Read the model definition and answer for the solid it produces. Units are mm, in the model's axes. A direction names the side the tool comes from. Round coordinates to 2 decimals unless told otherwise and drop trailing zeros. Write each loop counter-clockwise with the first axis right and the second up, starting at its lowest first coordinate (ties: lowest second). Pieces come first, ordered by that corner, then holes. Notation, with made-up numbers: (-30.5, 55) - (-8.5, 55) arc R26 cw to (-8.5, 94) - close; hole circle Ø3 at (55.5, 60.25). An arc over 180 degrees is marked (long way). One line per item, written item: value. Start each with the question number.
(1) A cutting plane is placed at A-A, the plane x = -27.8. Determine the outline of the cut face in (y, z).
(2) Find the intervals of material crossed by L1, parallel to X at y = 33, z = 96.5, in increasing order.
(3) For faces 1 (the face through (-27.76, 72.75, 2.54)), 2 (the face through (-18, 67, 5)), 3 (the face through (-18, 91, 5)), 4 (the face through (-5, 3, 179)), 5 (the face through (-5, 5, 91)), determine the directions among +Z, -Z, +X, -X, +Y, -Y from which every point of the face is accessible in a straight line to the end or side of a thin tool.
(4) A cutting plane is placed at C-C, the plane z = 120.5. Determine the outline of the cut face in (x, y).
(5) A cutting plane is placed at B-B, the plane x = -5. Determine the outline of the cut face in (y, z), plus the area to 3 significant figures.
(6) The mould has two halves that part along Y. Classify faces 6 (the face through (-10, 99, 3)), 7 (the face through (-3, 3, 175)), 8 (the face through (-29.55, 69, 3)): +Y half, -Y half, draft (parallel to the pull), parting line (faces both ways), or undercut.
(7) Flat-ended cylindrical pins translate along their axes: pin 1 Ø1.2 at (y, z) = (1.5, 58) entering from -X; pin 2 Ø8 at (x, z) = (-9, 80.5) entering from +Y; pin 3 Ø5 at (x, y) = (-19, 94.5) entering from +Z; pin 4 Ø12 at (x, z) = (-21.5, 145.5) entering from +Y. Find the tip coordinate at first contact, or state that the pin passes through.
(8) A cutting plane is placed at D-D, the plane x = -17. Determine the outline of the cut face in (y, z), plus the area to 3 significant figures.
from build123d import *

# Parameters (mm, degrees)
F0_W        = 54
F0_H        = 5
F0_W_2      = 40
F1_DEPTH    = 5
F2_DEPTH    = 10
F3_DEPTH    = 35
F5_DEPTH    = 5.001
F7_DEPTH    = 5.001
F4_W        = 35
F4_H        = 4
F8_DEPTH    = 40
F9_T4_DEPTH = 106.8673195186
F10_R       = 2
F11_R       = 10
F12_SIZE    = 0.6


# Not quite as in the source:
# - a fillet or chamfer that OpenCascade refuses, or shapes differently, is made with other operations: its cross-section is extruded or revolved along the edge and cut away or added


with BuildPart() as f1:
    # F0 (on Right) → F1 (new body)
    with BuildSketch(Plane.YZ):
        Polygon((0, 185), (0, 0), (5, 0), (5, 5), (5, 185), align=None)
        with Locations((32, 2.5)):
            Rectangle(F0_W, F0_H)
        Polygon((10, 185), (5, 185), (5, 5), (59, 5), (99, 5), (99, 10), align=None)
        with Locations((79, 2.5)):
            Rectangle(F0_W_2, F0_H)
    extrude(amount=F1_DEPTH)

    # F0 (on Right) → F2 (join)
    with BuildSketch(Plane.YZ):
        Polygon((0, 185), (0, 0), (5, 0), (5, 5), (5, 185), align=None)
    extrude(amount=-F2_DEPTH)

    # F0 (on Right) → F3 (join)
    with BuildSketch(Plane.YZ):
        with Locations((79, 2.5)):
            Rectangle(F0_W_2, F0_H)
    extrude(amount=-F3_DEPTH)

    # F4 (on face) → F5 (cut, through all)
    with BuildSketch(Plane.XY.offset(5)):
        with BuildLine():
            Line((-26.05, 69), (-26.05, 71))
            ThreePointArc((-26.05, 71), (-27.8, 72.75), (-29.55, 71))
            Line((-29.55, 71), (-29.55, 69))
            Line((-29.55, 69), (-29.55, 67))
            ThreePointArc((-29.55, 67), (-27.8, 65.25), (-26.05, 67))
            Line((-26.05, 67), (-26.05, 69))
        make_face()
        with BuildLine():
            Line((-26.05, 89), (-26.05, 91))
            ThreePointArc((-26.05, 91), (-27.8, 92.75), (-29.55, 91))
            Line((-29.55, 91), (-29.55, 89))
            Line((-29.55, 89), (-29.55, 87))
            ThreePointArc((-29.55, 87), (-27.8, 85.25), (-26.05, 87))
            Line((-26.05, 87), (-26.05, 89))
        make_face()
    extrude(amount=-F5_DEPTH, mode=Mode.SUBTRACT)

    # F6 (on face) → F7 (cut, through all)
    with BuildSketch(Plane(origin=(0, 5, 0), x_dir=(-1, 0, 0), z_dir=(0, 1, 0))):
        with BuildLine():
            Line((7, 58), (7, 60))
            ThreePointArc((7, 60), (5, 62), (3, 60))
            Line((3, 60), (3, 58))
            Line((3, 58), (3, 56))
            ThreePointArc((3, 56), (5, 54), (7, 56))
            Line((7, 56), (7, 58))
        make_face()
        with BuildLine():
            Line((7, 175), (7, 177))
            ThreePointArc((7, 177), (5, 179), (3, 177))
            Line((3, 177), (3, 175))
            Line((3, 175), (3, 173))
            ThreePointArc((3, 173), (5, 171), (7, 173))
            Line((7, 173), (7, 175))
        make_face()
    extrude(amount=-F7_DEPTH, mode=Mode.SUBTRACT)

    # F4 (on face) → F8 (join)
    with BuildSketch(Plane.XY.offset(5)):
        with Locations((-17.5, 79)):
            Rectangle(F4_W, F4_H)
    extrude(amount=F8_DEPTH)

    # F9: chamfer of 40 on 1 edges, made by hand


with BuildPart() as f9_tool2:
    # F9_s3 → F9_t4 (new body)
    with BuildSketch(Plane.XZ.offset(-183.8673195186)):
        Polygon((-35, 5), (5, 45), (-35, 45), align=None)
    extrude(amount=F9_T4_DEPTH)

    split(bisect_by=Plane.YZ, keep=Keep.BOTTOM)


with BuildPart() as f1_1:
    add(f1.part)

    # F9_t1: cut F9_tool2
    add(f9_tool2.part, mode=Mode.SUBTRACT)

    # F10
    f10_edges = [f1_1.edges().sort_by_distance(p)[0] for p in [
        (-17.5, 77, 5),
        (0, 77, 22.5),
        (0, 81, 22.5),
        (-17.5, 81, 5),
        (0, 68, 5),
        (0, 90, 5),
    ]]
    fillet(f10_edges, radius=F10_R)

    # F11
    f11_edges = [f1_1.edges().sort_by_distance(p)[0] for p in [
        (-35, 59, 2.5),
        (-35, 99, 2.5),
    ]]
    fillet(f11_edges, radius=F11_R)

    # F12
    f12_edges = [f1_1.edges().sort_by_distance(p)[0] for p in [
        (5, 0, 92.5),
        (5, 49.5, 0),
        (5, 99, 5),
        (5, 54.5, 97.5),
        (5, 5, 185),
    ]]
    chamfer(f12_edges, length=F12_SIZE)


solid = f1_1.part
Here are the results:
1. outline: (59.4, 0) - (65.25, 0) - (65.25, 5) - (59.4, 5) - close; (72.75, 0) - (85.25, 0) - (85.25, 5) - (83, 5) arc R2 cw to (81, 7) - (81, 12.2) - (77, 12.2) - (77, 7) arc R2 cw to (75, 5) - (72.75, 5) - close; (92.75, 0) - (98.6, 0) - (98.6, 5) - (92.75, 5) - close
2. L1: 0 to 5
3. face 1: +Z, -Z
3. face 2: +Z, -X
3. face 3: +Z, -X, +Y
3. face 4: +Y, -Y
3. face 5: +Z, -Z, -X
4. outline: (-10, 0) - (4.4, 0) - (5, 0.6) - (5, 42.13) - (4.4, 42.8) - (0, 42.8) - (0, 5) - (-10, 5) - close
5. outline: (0, 0) - (5, 0) - (5, 54) - (0, 54) - close; (0, 62) - (5, 62) - (5, 171) - (0, 171) - close; (0, 179) - (5, 179) - (5, 185) - (0, 185) - close; (59, 0) - (99, 0) - (99, 5) - (83, 5) arc R2 cw to (81, 7) - (81, 35) - (77, 35) - (77, 7) arc R2 cw to (75, 5) - (59, 5) - close
5. area: 1,170 mm²
6. face 6: +Y half
6. face 7: draft
6. face 8: undercut
7. pin 1: x = -10
7. pin 2: y = 5
7. pin 3: z = 5
7. pin 4: through
8. outline: (59, 0) - (99, 0) - (99, 5) - (83, 5) arc R2 cw to (81, 7) - (81, 23) - (77, 23) - (77, 7) arc R2 cw to (75, 5) - (59, 5) - close
8. area: 274 mm²
